from build123d import *

# Parameters (mm, degrees)
SKETCH_1_R          = 4
EXTRUDE_1_DEPTH     = 12
SKETCH_2_R          = 5.5
EXTRUDE_2_DEPTH     = 5
SKETCH_3_R          = 4
CUT_EXTRUDE_5_DEPTH = 2
SKETCH_5_R          = 1.5
CUT_EXTRUDE_6_DEPTH = 15.300349646


with BuildPart() as part:
    # 草图1 → 拉伸1 (new body)
    with BuildSketch(Plane.XY):
        Circle(SKETCH_1_R)
    extrude(amount=EXTRUDE_1_DEPTH)

    # 草图2 → 拉伸2 (add)
    with BuildSketch(Plane(origin=(0, 0, 0), x_dir=(-1, 0, 0), z_dir=(0, 0, -1))):
        Circle(SKETCH_2_R)
    extrude(amount=-EXTRUDE_2_DEPTH)

    # 草图3 → 拉伸5 (cut)
    with BuildSketch(Plane(origin=(0, 0, 0), x_dir=(-1, 0, 0), z_dir=(0, 0, -1))):
        Circle(SKETCH_3_R)
    extrude(amount=-CUT_EXTRUDE_5_DEPTH, mode=Mode.SUBTRACT)

    # 草图5 → 拉伸6 (cut, through all)
    with BuildSketch(Plane.XY.offset(12)):
        Circle(SKETCH_5_R)
    extrude(amount=-CUT_EXTRUDE_6_DEPTH, mode=Mode.SUBTRACT)


solid = part.part
Input: part model. Units: mm. Frame: model coordinates. A direction names the side the tool comes from. Give positions to 0.01 mm unless a question says otherwise; leave off trailing zeros. Order: outer loops, then holes, each group sorted by start corner. A loop starts at its lowest first (then second) coordinate and runs counter-clockwise, first axis right, second up. Notation, with made-up numbers: (-14.5, 36.25) - (-3.5, 36.25) arc R15 ccw to (-3.5, 53.25) - close; hole circle Ø6 at (-20, 48). An arc over 180 degrees is marked (long way). Answer as a JSON object with one key per item and string values. Group by question number.
Q1. Cut plane A-A, the plane x = 0. Output: boundary loops of the cut face in (y, z).
Q2. Cut plane D-D, the plane x = -3. Output: boundary loops of the cut face in (y, z), then the cut area to 3 significant figures.
Q3. Mould query, pull axis Y, two halves, no side actions, for faces 4 (the face through (-1.5, 0.07, 7.07)), 5 (the face through (4, -2, 0)), 6 (the face through (-2, 0, 2)), 7 (the face through (-0.867, -3.905, 8.451)). Classes: pulls with the +Y half, pulls with the -Y half, needs draft (parallel to the pull), parting line crosses it, or undercut.
Q4. Set-up query: faces 1 (the face through (4, -2, 5)), 2 (the face through (2, 0, 12)), 3 (the face through (0.867, -3.905, 0.986)). Return all of +Z, -Z, +X, -X, +Y, -Y with unobstructed straight access to the full face (end or side cutting, diameter ignored); none if empty.
Q5. Cut plane C-C, the plane z = 10.5. Output: boundary loops of the cut face in (x, y), then the cut area to 3 significant figures.
Q6. First-contact query: pin 1 Ø4 at (x, z) = (2.5, 4) entering from +Y; pin 2 Ø6 at (y, z) = (-3.5, 5.5) entering from +X; pin 3 Ø1 at (y, z) = (-3, 4.5) entering from -X. Flat tips, straight axial feed; report the tip coordinate or a pass-through.
Q7. Line query: probe 1 along Y at (x, z) = (0, 0.6); probe 2 along Y at (x, z) = (0, 8.25); probe 3 along Z at (x, y) = (-2.5, 4). Output: solid intervals per line, ascending.
Results:
{
 "1": {"outline": "(-5.5, 0) - (-4, 0) - (-4, 2) - (-1.5, 2) - (-1.5, 12) - (-4, 12) - (-4, 5) - (-5.5, 5) - close; (1.5, 2) - (4, 2) - (4, 0) - (5.5, 0) - (5.5, 5) - (4, 5) - (4, 12) - (1.5, 12) - close"},
 "2": {"outline": "(-4.61, 0) - (-2.65, 0) - (-2.65, 2) - (2.65, 2) - (2.65, 0) - (4.61, 0) - (4.61, 5) - (2.65, 5) - (2.65, 12) - (-2.65, 12) - (-2.65, 5) - (-4.61, 5) - close", "area": "72.6 mm^2"},
 "3": {"face 4": "undercut", "face 5": "needs draft", "face 6": "undercut", "face 7": "parting line crosses it"},
 "4": {"face 1": "+Z", "face 2": "+Z, +X, -X, +Y, -Y", "face 3": "-Z"},
 "5": {"outline": "circle Ø8 at (0, 0); hole circle Ø3 at (0, 0)", "area": "43.2 mm^2"},
 "6": {"pin 1": "y = 5.48", "pin 2": "x = 5.47", "pin 3": "x = -4.9"},
 "7": {"probe 1": "-5.5 to -4, 4 to 5.5", "probe 2": "-4 to -1.5, 1.5 to 4", "probe 3": "0 to 5"}
}
